Model file for the job. Use its own axes, mm. A direction names the side the tool comes from. Give positions to 0.01 mm unless a question says otherwise; leave off trailing zeros. Order: outer loops, then holes, each group sorted by start corner. A loop starts at its lowest first (then second) coordinate and runs counter-clockwise, first axis right, second up. Notation, with made-up numbers: M -23.5,-1 L 16.5,-1 A22 ccw 16.5,9 Z; hole C 25.5,21.25 d5. An arc over 180 degrees is marked long. Return JSON: item names as keys, results as strings. Group by question number.
1. 3-axis set-ups, long thin cutter, end or side, ignore diameter. For faces 1 (the face through (57, 52, 12)), 2 (the face through (44, 26, 18)), 3 (the face through (20, 36, 41)), 4 (the face through (57, 0, 12)), 5 (the face through (-20, 16, 41)): which of +Z, -Z, +X, -X, +Y, -Y reach the whole face in a straight line?
2. Pin check, flat tips, straight feed: pin 1 (8 mm diameter, centred on x = 21, z = 38.5, fed in from +Y); pin 2 (16.5 mm diameter, centred on x = 68.5, z = 14.5, fed in from -Y); pin 3 (16 mm diameter, centred on x = 81, y = 29, fed in from +Z). Stop position of each tip, or through.
3. Slice it at A-A on x = 0. List the corners of the cut face in (y, z), then the cut area to 3 significant figures.
4. Slice it at C-C on y = 26. List the corners of the cut face in (x, z), then the cut area to 3 significant figures.
5. Wall check: probe 1 along X at (y, z) = (26, 12.5); probe 2 along Y at (x, z) = (0, 14); probe 3 along Y at (x, z) = (87, 18). Give the ranges that are in metal, low to high. Write a range as [from, to].
6. Slice it at D-D on x = 45.5. List the corners of the cut face in (y, z), then the cut area to 3 significant figures.
7. Slice it at B-B on z = 16.5. List the corners of the cut face in (x, y).
8. Two-plate mould, pull along X, no slides. Class faces 6 (the face through (72, 42, 18)), 7 (the face through (91, 5, 20)), 8 (the face through (7.055, 11.639, 19.794)): released by +X, released by -X, zero draft, split by the parting line, or undercut.
from build123d import *

# Parameters (mm, degrees)
SKETCH1_W           = 100
SKETCH1_H           = 52
BOSS_EXTRUDE1_DEPTH = 25
SKETCH2_R           = 30
BOSS_EXTRUDE2_DEPTH = 50
CUT_EXTRUDE1_REACH  = 127.044
SKETCH4_W           = 56
SKETCH4_H           = 32
CUT_EXTRUDE2_DEPTH  = 15
SKETCH5_OUTSIDE_W   = 162.332
SKETCH5_OUTSIDE_H   = 92.332
SKETCH5_OUTSIDE_W_2 = 73.851546866
SKETCH5_OUTSIDE_H_2 = 20
CUT_EXTRUDE3_DEPTH  = 18
CUT_EXTRUDE4_REACH  = 127.044
SKETCH6_R           = 16


with BuildPart() as part:
    # Sketch1 → Boss-Extrude1 (new body)
    with BuildSketch(Plane.XY):
        with Locations((50, 26)):
            Rectangle(SKETCH1_W, SKETCH1_H)
    extrude(amount=BOSS_EXTRUDE1_DEPTH)

    # Sketch2 → Boss-Extrude2 (add)
    with BuildSketch(Plane(origin=(0, 0, 0), x_dir=(-1, 0, 0), z_dir=(0, 0, -1))):
        with Locations((0, 26)):
            Circle(SKETCH2_R)
    extrude(amount=-BOSS_EXTRUDE2_DEPTH)

    # Sketch3 → Cut-Extrude1 (cut, up to next)
    with BuildSketch(Plane(origin=(0, 52, 0), x_dir=(1, 0, 0), z_dir=(0, 1, 0)), mode=Mode.PRIVATE) as cut_extrude1_sk1:
        Polygon((100, -25), (100, -15), (82, -25), align=None)
    cut_extrude1_tool1 = extrude(cut_extrude1_sk1.sketch, amount=-CUT_EXTRUDE1_REACH, mode=Mode.PRIVATE) & part.part
    add(cut_extrude1_tool1.solids().sort_by_distance((94, 52, 21.666667))[0], mode=Mode.SUBTRACT)

    # Sketch4 → Cut-Extrude2 (cut)
    with BuildSketch(Plane.XY.offset(25)):
        with Locations((72, 26)):
            Rectangle(SKETCH4_W, SKETCH4_H)
    extrude(amount=-CUT_EXTRUDE2_DEPTH, mode=Mode.SUBTRACT)

    # Sketch5 outside → Cut-Extrude3 (cut)
    with BuildSketch(Plane.XY.offset(50)):
        with Locations((35, 26)):
            Rectangle(SKETCH5_OUTSIDE_W, SKETCH5_OUTSIDE_H)
        with Locations((0, 26)):
            Rectangle(SKETCH5_OUTSIDE_W_2, SKETCH5_OUTSIDE_H_2, mode=Mode.SUBTRACT)
    extrude(amount=-CUT_EXTRUDE3_DEPTH, mode=Mode.SUBTRACT)

    # Sketch6 → Cut-Extrude4 (cut, up to next)
    with BuildSketch(Plane.XY.offset(50), mode=Mode.PRIVATE) as cut_extrude4_sk1:
        with Locations(Location((0, 26, 0), (0, 0, 38.682187453))):
            Circle(SKETCH6_R)
    cut_extrude4_tool1 = extrude(cut_extrude4_sk1.sketch, amount=-CUT_EXTRUDE4_REACH, mode=Mode.PRIVATE) & part.part
    add(cut_extrude4_tool1.solids().sort_by_distance((0, 26, 50))[0], mode=Mode.SUBTRACT)


solid = part.part
Result:
{
 "1": {"face 1": "+Z, -Z, +X, +Y", "face 2": "+Z, +X", "face 3": "+Z, +X, -X, +Y", "face 4": "+Z, -Z, +X, -Y", "face 5": "+Z, +X, -X, -Y"},
 "2": {"pin 1": "stops at y = 36", "pin 2": "stops at y = 0", "pin 3": "stops at z = 10"},
 "3": {"outline": "M -4,0 L 10,0 L 10,32 L -4,32 Z; M 42,0 L 56,0 L 56,32 L 42,32 Z", "area": "896 mm2"},
 "4": {"outline": "M -30,0 L -16,0 L -16,50 L -30,50 Z; M 16,0 L 100,0 L 100,10 L 44,10 L 44,25 L 30,25 L 30,50 L 16,50 Z", "area": "2,310 mm2"},
 "5": {"probe 1": "x = [-30, -16], [16, 44]", "probe 2": "y = [-4, 10], [42, 56]", "probe 3": "y = [0, 10], [42, 52]"},
 "6": {"outline": "M 0,0 L 52,0 L 52,25 L 42,25 L 42,10 L 10,10 L 10,25 L 0,25 Z", "area": "820 mm2"},
 "7": {"outline": "M 14.97,0 L 97.3,0 L 97.3,10 L 44,10 L 44,42 L 97.3,42 L 97.3,52 L 14.97,52 A30 ccw long Z; hole C 0,26 d32"},
 "8": {"face 6": "zero draft", "face 7": "released by +X", "face 8": "undercut"}
}
